Here's how the part is built. I have some questions about the finished solid (model axes, mm). A direction names the side the tool comes from. Coordinates: 2 decimals unless noted, no trailing zeros. Write each loop counter-clockwise with the first axis right and the second up, starting at its lowest first coordinate (ties: lowest second). Pieces come first, ordered by that corner, then holes.
Item 1: If we mould it in two halves opening along Y, with no side actions, what happens to faces 1 (the face through (4, 3, 84)), 2 (the face through (2, 5, 0)), 3 (the face through (1.014, 15.535, 81.095)), 4 (the face through (12, 0, 84))? For each: pulls with the +Y half, pulls with the -Y half, needs draft (parallel to the pull), parting line crosses it, or undercut.
Item 2: For faces 5 (the face through (0, 10, 84)), 6 (the face through (16, 2, 84)), which set-ups out of +Z, -Z, +X, -X, +Y, -Y let a thin tool reach every point of the face, with its end or its side?
Item 3: Please list where these lines run through material, in increasing order: line 1 (X direction, y = 14, z = 151.5); line 2 (X direction, y = 1.75, z = 110).
Item 4: I want a section at B-B (y = 15.25). Please give me the cut outline in (x, z).
Item 5: I'm going to push flat-ended pins straight in: P1, Ø8.5, axis at x = 15.5, z = 87.5, coming from the +Y side; P2, Ø6, axis at y = 19, z = 100, coming from the +X side; P3, Ø3, axis at y = 6, z = 32, coming from the +X side. Where does each tip first touch, or does it pass through?
Item 6: I want a section at D-D (y = 22). Please give me the cut outline in (x, z).
from build123d import *

# Parameters (mm, degrees)
EXTRUDE_1_DEPTH     = 170
FILLET_1_R          = 1
SKETCH_2_R          = 4
CUT_EXTRUDE_1_DEPTH = 174.360895245


with BuildPart() as part:
    # 草图1 → 凸台-拉伸1 (new body)
    with BuildSketch(Plane.XY):
        with BuildLine():
            Line((0, 0), (25, 0))
            Line((25, 0), (25, 2))
            Line((25, 2), (7, 2))
            ThreePointArc((7, 2), (3.464466094, 3.464466094), (2, 7))
            Line((2, 7), (2, 25))
            Line((2, 25), (0, 25))
            Line((0, 25), (0, 0))
        make_face()
    extrude(amount=EXTRUDE_1_DEPTH)

    # 圆角1
    fillet_1_edges = [part.edges().sort_by_distance(p)[0] for p in [
        (0, 25, 85),
        (25, 2, 85),
        (25, 0, 85),
        (0, 0, 85),
        (2, 25, 85),
    ]]
    fillet(fillet_1_edges, radius=FILLET_1_R - 0.0001)  # a hair under: the kernel refuses the full size

    # 草图2 → 切除-拉伸1 (cut, through all)
    with BuildSketch(Plane(origin=(2, 0, 0), x_dir=(0, 0, -1), z_dir=(1, 0, 0))):
        with Locations(Location((-85, 16.401885755, 0), (0, 0, 90))):
            Circle(SKETCH_2_R)
    extrude(amount=-CUT_EXTRUDE_1_DEPTH, mode=Mode.SUBTRACT)


solid = part.part
Answer:
1. face 1: pulls with the +Y half
1. face 2: needs draft
1. face 3: undercut
1. face 4: pulls with the -Y half
2. face 5: +Z, -Z, -X, +Y, -Y
2. face 6: +Z, -Z, +X, +Y
3. line 1: x = 0 to 2
3. line 2: x = 0 to 24.66
4. outline: (0, 0) - (2, 0) - (2, 81.17) - (0, 81.17) - close; (0, 88.83) - (2, 88.83) - (2, 170) - (0, 170) - close
5. P1: stops at y = 2
5. P2: stops at x = 2
5. P3: stops at x = 2.67
6. outline: (0, 0) - (2, 0) - (2, 170) - (0, 170) - close
